from build123d import *

# Parameters (mm, degrees)
SKETCH_1_R          = 6
EXTRUDE_1_DEPTH     = 5
SKETCH_2_W          = 12
SKETCH_2_H          = 8
EXTRUDE_2_DEPTH     = 6
SKETCH_2_2_W        = 12
SKETCH_2_2_H        = 8
EXTRUDE_3_DEPTH     = 6
SKETCH_3_R          = 2
CUT_EXTRUDE_1_DEPTH = 16.620499352
SKETCH_4_R          = 1.5
CUT_EXTRUDE_2_DEPTH = 5
FILLET_1_R          = 2
SKETCH_5_R          = 3
CUT_EXTRUDE_4_DEPTH = 2.6


with BuildPart() as part:
    # Sketch 1 → Extrude 1 (new body)
    with BuildSketch(Plane(origin=(0, 0, 0), x_dir=(1, 0, 0), z_dir=(0, 1, 0))):
        with Locations(Location((0, 0, 0), (0, 0, 270))):
            Circle(SKETCH_1_R)
    extrude(amount=EXTRUDE_1_DEPTH)

    # Sketch 2 → Extrude 2 (add)
    with BuildSketch(Plane.XY):
        with Locations((0, -4)):
            Rectangle(SKETCH_2_W, SKETCH_2_H)
    extrude(amount=-EXTRUDE_2_DEPTH)

    # Sketch 2_2 → Extrude 3 (add)
    with BuildSketch(Plane.XY):
        with Locations((0, -4)):
            Rectangle(SKETCH_2_2_W, SKETCH_2_2_H)
    extrude(amount=EXTRUDE_3_DEPTH)

    # Sketch 3 → Cut-Extrude 1 (cut, through all)
    with BuildSketch(Plane.XY.offset(6)):
        with Locations((0, -4)):
            Circle(SKETCH_3_R)
    extrude(amount=-CUT_EXTRUDE_1_DEPTH, mode=Mode.SUBTRACT)

    # Sketch 4 → Cut-Extrude 2 (cut)
    with BuildSketch(Plane(origin=(0, 5, 0), x_dir=(1, 0, 0), z_dir=(0, 1, 0))):
        with Locations(Location((0, 0, 0), (0, 0, 270))):
            Circle(SKETCH_4_R)
    extrude(amount=-CUT_EXTRUDE_2_DEPTH, mode=Mode.SUBTRACT)

    # Fillet 1
    fillet_1_edges = [part.edges().sort_by_distance(p)[0] for p in [
        (-6, -4, 6),
        (6, -4, 6),
        (-6, -4, -6),
        (6, -4, -6),
    ]]
    fillet(fillet_1_edges, radius=FILLET_1_R)

    # Sketch 5 → Cut-Extrude 4 (cut)
    with BuildSketch(Plane(origin=(0, 5, 0), x_dir=(1, 0, 0), z_dir=(0, 1, 0))):
        with Locations(Location((0, 0, 0), (0, 0, 270))):
            Circle(SKETCH_5_R)
    extrude(amount=-CUT_EXTRUDE_4_DEPTH, mode=Mode.SUBTRACT)


solid = part.part
Geometry check sheet. Reference: the model listing, model coordinates, mm. A direction names the side the tool comes from. Round coordinates to 2 decimals unless told otherwise and drop trailing zeros. Loops run counter-clockwise (first coordinate to the right, second up) from the corner with the lowest first, then second, coordinate; pieces in that order, holes last.
Item 1: Cross-section at D-D on y = -1.5. Record the boundary of the cut face in (x, z), then the cut area to 3 significant figures.
Item 2: Mould release check, pull along X, two halves, no side actions. Record for faces 5 (the flat face through (6, -4, 0)), 6 (the cylindrical face through (0, -6, 0)), 7 (the flat face through (5, 0, -5)): pulls with the +X half, pulls with the -X half, needs draft (parallel to the pull), parting line crosses it, or undercut.
Item 3: Cross-section at C-C on z = -3.5. Record the boundary of the cut face in (x, y).
Item 4: Cross-section at B-B on x = 1. Record the boundary of the cut face in (y, z).
Item 5: Access from +Z, -Z, +X, -X, +Y, -Y to the whole of each face (thin tool, end or side, straight path). Record for faces 1 (the flat face through (0, 0, 0)), 2 (the flat face through (-5, 0, 5)), 3 (the cylindrical face through (-5.43, -3.94, 5.4)), 4 (the flat face through (-5, 0, -5)).
Item 6: Thickness scan on line 1 (Y direction, x = 0, z = 0.75); line 2 (X direction, y = 3.4, z = 0); line 3 (Y direction, x = 2.5, z = 0.75). Record the ranges inside material, lowest first.
Item 7: Gauge pin test, flat ends, axial feed: pin 1 (2 mm diameter, centred on x = 4.5, y = -2, fed in from +Z); pin 2 (3 mm diameter, centred on x = 1, z = -0.5, fed in from +Y); pin 3 (2.5 mm diameter, centred on x = 0, z = 0, fed in from +Y); pin 4 (1 mm diameter, centred on y = 3, z = -2.5, fed in from +X). Record the tip position at first contact, or that the pin passes through.
Item 8: Cross-section at A-A on y = -4. Record the boundary of the cut face in (x, z).
Answer sheet:
1. outline: (-6, -4) arc R2 ccw to (-4, -6) - (4, -6) arc R2 ccw to (6, -4) - (6, 4) arc R2 ccw to (4, 6) - (-4, 6) arc R2 ccw to (-6, 4) - close
1. area: 141 mm2
2. face 5: pulls with the +X half
2. face 6: undercut
2. face 7: needs draft
3. outline: (-6, -8) - (6, -8) - (6, 0) - (4.87, 0) - (4.87, 5) - (-4.87, 5) - (-4.87, 0) - (-6, 0) - close; hole circle Ø4 at (0, -4)
4. outline: (-8, -6) - (-5.73, -6) - (-5.73, 6) - (-8, 6) - close; (-2.27, -6) - (0, -6) - (0, -5.92) - (5, -5.92) - (5, -2.83) - (2.4, -2.83) - (2.4, -1.12) - (0, -1.12) - (0, 1.12) - (2.4, 1.12) - (2.4, 2.83) - (5, 2.83) - (5, 5.92) - (0, 5.92) - (0, 6) - (-2.27, 6) - close
5. face 1: +Y
5. face 2: +Z, -X, +Y
5. face 3: +Z, -X, +Y, -Y
5. face 4: -Z, -X, +Y
6. line 1: y = -8 to -6, -2 to 0
6. line 2: x = -6 to -3, 3 to 6
6. line 3: y = -8 to 2.4
7. pin 1: stops at z = 6
7. pin 2: stops at y = 2.4
7. pin 3: stops at y = 0
7. pin 4: stops at x = 5.66
8. outline: (-6, -4) arc R2 ccw to (-4, -6) - (-2, -6) - (-2, 6) - (-4, 6) arc R2 ccw to (-6, 4) - close; (2, -6) - (4, -6) arc R2 ccw to (6, -4) - (6, 4) arc R2 ccw to (4, 6) - (2, 6) - close
